Input: part model. Units: mm. Frame: model coordinates. A direction names the side the tool comes from. Give positions to 0.01 mm unless a question says otherwise; leave off trailing zeros. Loops run counter-clockwise (first coordinate to the right, second up) from the corner with the lowest first, then second, coordinate; pieces in that order, holes last. Notation, with made-up numbers: (28, -21.5) -> (86, -21.5) arc R8 cw to (86, -7.5) -> close; hole circle Ø3 at (68.5, 38). An arc over 180 degrees is marked (long way). One line per question, with ' | ' between items.
from build123d import *

# Parameters (mm, degrees)
F0_R     = 2.5
F1_DEPTH = 5
F2_SIZE  = 4.99999
F3_SIZE  = 2


# Not quite as in the source:
# - a fillet or chamfer is up to 0.001 mm smaller than in the source, because OpenCascade refuses the exact size


with BuildPart() as f1:
    # F0 (on Top) → F1 (new body)
    with BuildSketch(Plane.XY):
        Polygon((-5, 70), (-25, 70), (-25, 5), (-20, 0), (-25, -5), (-25, -60), (-5, -60), (0, -55), (5, -60), (25, -60), (25, -5), (20, 0), (25, 5), (25, 70), (5, 70), (0, 65), align=None)
        with Locations((-4.9999998882, -39)):
            Circle(F0_R, mode=Mode.SUBTRACT)
        Circle(F0_R, mode=Mode.SUBTRACT)
        with Locations((6, 26)):
            Circle(F0_R, mode=Mode.SUBTRACT)
        with Locations((0, 52)):
            Circle(F0_R, mode=Mode.SUBTRACT)
    extrude(amount=F1_DEPTH)

    # F2 (size 5 in the source; OpenCascade refuses exactly that, so slightly less here)
    f2_edges = [f1.edges().sort_by_distance(p)[0] for p in [
        (-2.5, 67.5, 5),
        (2.5, 67.5, 5),
        (22.5, 2.5, 5),
        (22.5, -2.5, 5),
        (-22.5, 2.5, 5),
        (-22.5, -2.5, 5),
        (-2.5, -57.5, 5),
        (2.5, -57.5, 5),
    ]]
    chamfer(f2_edges, length=F2_SIZE)

    # F3
    f3_edges = [f1.edges().sort_by_distance(p)[0] for p in [
        (-2.5, 52, 5),
        (3.5, 26, 5),
        (-7.5, -39, 5),
        (-2.5, 0, 5),
    ]]
    chamfer(f3_edges, length=F3_SIZE)


solid = f1.part
1. Section query A-A (y = 26). Output: boundary loops of the cut face in (x, z), then the cut area to 3 significant figures.
Determined:
outline: (-25, 0) -> (3.5, 0) -> (3.5, 3) -> (1.5, 5) -> (-25, 5) -> close; (8.5, 0) -> (25, 0) -> (25, 5) -> (10.5, 5) -> (8.5, 3) -> close | area: 221 mm2
2. Ray query, line 1 along Y through (x, z) = (0, 0.7); line 2 along Y through (x, z) = (-1, 1.1); line 3 along Y through (x, z) = (20.5, 2.65). Return the intervals inside material, ascending. Write a range as from..to.
Determined:
line 1: y = -54.01..-2.5, 2.5..49.5, 54.5..64.01 | line 2: y = -54.44..-2.29, 2.29..49.71, 54.29..64.44 | line 3: y = -60..-4.25, 4.25..70
3. Section query B-B (y = 9.5). Output: boundary loops of the cut face in (x, z).
Determined:
outline: (-25, 0) -> (25, 0) -> (25, 3.18) -> (22.43, 5) -> (-22.43, 5) -> (-25, 3.18) -> close
4. Pull-direction query (Y, two-part tool) for faces 6 (the flat face through (-17, -60, 2)), 7 (the flat face through (-25, 38, 2)), 8 (the cylindrical face through (7.34, 28.11, 1.48)); classes: pulls with the +Y half, pulls with the -Y half, needs draft (parallel to the pull), parting line crosses it, or undercut.
Determined:
face 6: pulls with the -Y half | face 7: needs draft | face 8: undercut
5. Pin query (flat end, axial travel): P1, Ø6.5, axis at x = -5, y = -39, coming from the +Z side; P2, Ø3, axis at x = -1, y = 38.5, coming from the -Z side. Return the tip coordinate at first contact, or that it passes through.
Determined:
P1: stops at z = 3.75 | P2: stops at z = 0
6. Reachability of faces 1 (the flat face through (17, -60, 2)), 2 (the flat face through (-4.6, 65.23, 3.09)), 3 (the flat face through (20.23, 4.6, 3.09)), 4 (the cylindrical face through (-0.54, -2.44, 1.48)), 5 (the flat face through (-20.23, -4.6, 3.09)) from +Z, -Z, +X, -X, +Y, -Y: full face, straight path, thin tool, end or side. Return the list, or none.
Determined:
face 1: +Z, -Z, +X, -X, -Y | face 2: +Z, +Y | face 3: +Z, +X | face 4: +Z, -Z | face 5: +Z, -X
